Verification items for this drawing (mm, ordinates from the low corner). A direction names the side the tool comes from. Round coordinates to 2 decimals unless told otherwise and drop trailing zeros. Loops run counter-clockwise (first coordinate to the right, second up) from the corner with the lowest first, then second, coordinate; pieces in that order, holes last. Notation, with made-up numbers: M 1,83.25 L 37,83.25 A7 cw 37,87.25 Z; hole C -33,-19 d9. An arc over 180 degrees is marked long. One line per item, written item: value.
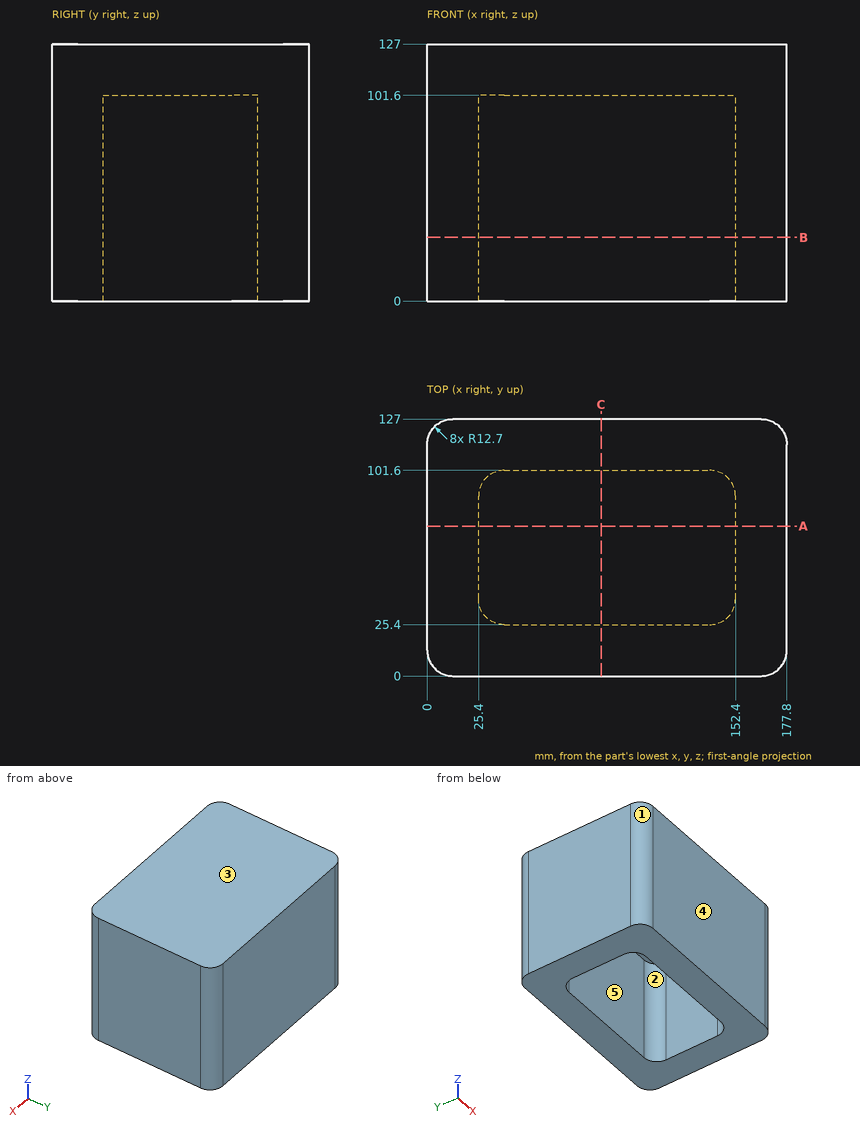
(1) Sectioned sample at A-A on y = 74. Enter the section's corners in (x, z).
Completed:
outline: M 0,0 L 25.4,0 L 25.4,101.6 L 152.4,101.6 L 152.4,0 L 177.8,0 L 177.8,127 L 0,127 Z
(2) Mould release check, pull along Y, two halves, no side actions. Record for the marked faces 3, 4 and 5: +Y half, -Y half, draft (parallel to the pull), parting line (faces both ways), or undercut.
Completed:
face 3: draft
face 4: -Y half
face 5: undercut
(3) Sectioned sample at C-C on x = 86. Enter the section's corners in (y, z), and give its area (3 significant figures).
Completed:
outline: M 0,0 L 25.4,0 L 25.4,101.6 L 101.6,101.6 L 101.6,0 L 127,0 L 127,127 L 0,127 Z
area: 8,390 mm^2
(4) Sectioned sample at B-B on z = 31.5. Enter the section's corners in (x, y).
Completed:
outline: M 0,12.7 A12.7 ccw 12.7,0 L 165.1,0 A12.7 ccw 177.8,12.7 L 177.8,114.3 A12.7 ccw 165.1,127 L 12.7,127 A12.7 ccw 0,114.3 Z; hole M 25.4,38.1 A12.7 ccw 38.1,25.4 L 139.7,25.4 A12.7 ccw 152.4,38.1 L 152.4,88.9 A12.7 ccw 139.7,101.6 L 38.1,101.6 A12.7 ccw 25.4,88.9 Z
(5) Tool access check on the marked faces 1 and 2. Record the directions out of +Z, -Z, +X, -X, +Y, -Y that give a thin tool (end or side, any length) a straight path to the whole face; none if there is none.
Completed:
face 1: +Z, -Z, -X, -Y
face 2: -Z
(6) Thickness scan on L1, parallel to Y at x = 79.5, z = 24.5; L2, parallel to X at y = 40.5, z = 22; L3, parallel to Z at x = 141, y = 53. Record the ranges inside material, lowest first. Write a range as from..to.
Completed:
L1: y = 0..25.4, 101.6..127
L2: x = 0..25.4, 152.4..177.8
L3: z = 101.6..127
